from build123d import *

# Parameters (mm, degrees)
SKETCH1_R           = 1.8
BOSS_EXTRUDE2_DEPTH = 5


with BuildPart() as part:
    # Sketch1 → Boss-Extrude2 (new body)
    # profile 1 of 2: a face of its own
    with BuildSketch(Plane.XY):
        with BuildLine():
            ThreePointArc((0, 9), (0.878679656, 11.121320344), (3, 12))
            Line((3, 12), (50, 12))
            Line((50, 12), (50, 0))
            Line((50, 0), (3, 0))
            ThreePointArc((3, 0), (0.878679656, 0.878679656), (0, 3))
            Line((0, 3), (0, 9))
        make_face()
        with Locations((6, 6)):
            Circle(SKETCH1_R, mode=Mode.SUBTRACT)
    # profile 2 of 2: a face of its own
    with BuildSketch(Plane.XY):
        with BuildLine():
            Line((90, -9), (69.8490214, -9))
            ThreePointArc((69.8490214, -9), (62.990773359, -6.428332012), (59.996714309, 0.256326008))
            Line((59.996714309, 0.256326008), (59.996714309, 11.743673992))
            ThreePointArc((59.996714309, 11.743673992), (62.990773359, 18.428332012), (69.8490214, 21))
            Line((69.8490214, 21), (90, 21))
            Line((90, 21), (90, 31))
            Line((90, 31), (70, 31))
            ThreePointArc((70, 31), (56.064971157, 25.642135624), (50, 12))
            Line((50, 12), (50, 0))
            ThreePointArc((50, 0), (56.064971157, -13.642135624), (70, -19))
            Line((70, -19), (90, -19))
            Line((90, -19), (90, -9))
        make_face()
    extrude(amount=BOSS_EXTRUDE2_DEPTH)


solid = part.part
Geometry check sheet. Reference: the model listing, model coordinates, mm. A direction names the side the tool comes from. Give positions to 0.01 mm unless a question says otherwise; leave off trailing zeros. Order: outer loops, then holes, each group sorted by start corner. A loop starts at its lowest first (then second) coordinate and runs counter-clockwise, first axis right, second up. Notation, with made-up numbers: (50, 75) - (68, 75) arc R19 cw to (68, 94) - close; hole circle Ø5 at (3, 7). An arc over 180 degrees is marked (long way). Use one line per item in the form item = value.
1) Material ranges on probe 1 along Y at (x, z) = (80, 3.85); probe 2 along Y at (x, z) = (6, 3.6); probe 3 along Y at (x, z) = (19, 0.7), recorded low to high. Write a range as from..to.
Working result:
probe_1 = -19..-9, 21..31
probe_2 = 0..4.2, 7.8..12
probe_3 = 0..12
2) Sectioned sample at C-C (y = 6). Record the boundary of the cut face in (x, z), and give its area (3 significant figures).
Working result:
outline = (0, 0) - (4.2, 0) - (4.2, 5) - (0, 5) - close; (7.8, 0) - (60, 0) - (60, 5) - (7.8, 5) - close
area = 282 mm^2
3) Sectioned sample at B-B (z = 4). Record the boundary of the cut face in (x, y), and give its area (3 significant figures).
Working result:
outline = (0, 3) arc R3 ccw to (3, 0) - (50, 0) arc R19.51 ccw to (70, -19) - (90, -19) - (90, -9) - (69.85, -9) arc R9.51 cw to (60, 0.26) - (60, 11.74) arc R9.51 cw to (69.85, 21) - (90, 21) - (90, 31) - (70, 31) arc R19.51 ccw to (50, 12) - (3, 12) arc R3 ccw to (0, 9) - close; hole circle Ø3.6 at (6, 6)
area = 1,560 mm^2
4) Draft check along Y on faces 4 (the face through (0.86, 11.1, 2.46)), 5 (the face through (54, 6, 0)), 6 (the face through (80, -9, 2)). Enter one of: released by +Y, released by -Y, zero draft, split by the parting line, or undercut.
Working result:
face_4 = released by +Y
face_5 = zero draft
face_6 = undercut
5) Access from +Z, -Z, +X, -X, +Y, -Y to the whole of each face (thin tool, end or side, straight path). Record for faces 1 (the face through (59.997, 6, 2)), 2 (the face through (6.831, 4.403, 2.465)), 3 (the face through (26, 12, 2)).
Working result:
face_1 = +Z, -Z, +X
face_2 = +Z, -Z
face_3 = +Z, -Z, -X, +Y
6) Depth check by flat-ended pin: pin 1 Ø2 at (x, z) = (79.5, 1) entering from -Y; pin 2 Ø2.5 at (x, z) = (80.5, 3) entering from +Y; pin 3 Ø1 at (y, z) = (-0.5, 4.5) entering from +X. Enter the tip coordinate at first touch or a pass-through.
Working result:
pin_1 = -19
pin_2 = 31
pin_3 = 60.11
7) Sectioned sample at D-D (x = 19). Record the boundary of the cut face in (y, z).
Working result:
outline = (0, 0) - (12, 0) - (12, 5) - (0, 5) - close
8) Sectioned sample at A-A (x = 6). Record the boundary of the cut face in (y, z).
Working result:
outline = (0, 0) - (4.2, 0) - (4.2, 5) - (0, 5) - close; (7.8, 0) - (12, 0) - (12, 5) - (7.8, 5) - close
